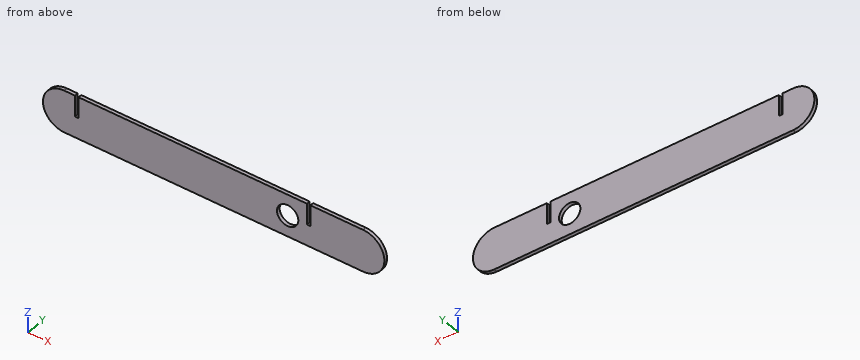
```python
from build123d import *

# Parameters (mm, degrees)
F0_R     = 4.7625
F1_DEPTH = 1.5875


with BuildPart() as f1:
    # F0 (on Front) → F1 (new body)
    with BuildSketch(Plane.XZ):
        with BuildLine():
            Line((-66.675, -9.525), (66.675, -9.525))
            ThreePointArc((66.675, -9.525), (76.2, 0), (66.675, 9.525))
            Line((66.675, 9.525), (43.18, 9.525))
            Line((43.18, 9.525), (43.18, 0))
            Line((43.18, 0), (41.5925, 0))
            Line((41.5925, 0), (41.5925, 9.525))
            Line((41.5925, 9.525), (-60.325, 9.525))
            Line((-60.325, 9.525), (-60.325, 0))
            Line((-60.325, 0), (-61.9125, 0))
            Line((-61.9125, 0), (-61.9125, 9.525))
            Line((-61.9125, 9.525), (-66.675, 9.525))
            ThreePointArc((-66.675, 9.525), (-76.2, 0), (-66.675, -9.525))
        make_face()
        with Locations((33.02, 0)):
            Circle(F0_R, mode=Mode.SUBTRACT)
    extrude(amount=F1_DEPTH)


solid = f1.part
```
Geometry check sheet. Reference: the model listing, model coordinates, mm. Give positions to 0.01 mm unless a question says otherwise; leave off trailing zeros. Write each loop counter-clockwise with the first axis right and the second up, starting at its lowest first coordinate (ties: lowest second). Pieces come first, ordered by that corner, then holes. Notation, with made-up numbers: (83.25, 4) -> (114.25, 4) arc R32 cw to (114.25, 43) -> close; hole circle Ø10 at (12, 46). An arc over 180 degrees is marked (long way). One line per question, with ' | ' between items.
Item 1: Depth check by flat-ended pin: pin 1 (0.8 mm diameter, centred on y = -1, z = 4, fed in from -X); pin 2 (6 mm diameter, centred on x = -16, z = -7.5, fed in from +Y); pin 3 (0.5 mm diameter, centred on x = -61, y = -0.5, fed in from +Z); pin 4 (0.8 mm diameter, centred on y = -0.5, z = 3.5, fed in from +X). Enter the tip coordinate at first touch or a pass-through.
Determined:
pin 1: x = -75.49 | pin 2: y = 0 | pin 3: z = 0 | pin 4: x = 75.68
Item 2: Sectioned sample at D-D, the plane z = 8.25. Record the boundary of the cut face in (x, y) (1 decimal), plus the area to 3 significant figures.
Determined:
outline: (-71.4, -1.6) -> (-61.9, -1.6) -> (-61.9, 0) -> (-71.4, 0) -> close; (-60.3, -1.6) -> (41.6, -1.6) -> (41.6, 0) -> (-60.3, 0) -> close; (43.2, -1.6) -> (71.4, -1.6) -> (71.4, 0) -> (43.2, 0) -> close | area: 222 mm^2
Item 3: Sectioned sample at B-B, the plane z = 2.5. Record the boundary of the cut face in (x, y) (1 decimal), plus the area to 3 significant figures.
Determined:
outline: (-75.9, -1.6) -> (-61.9, -1.6) -> (-61.9, 0) -> (-75.9, 0) -> close; (-60.3, -1.6) -> (29, -1.6) -> (29, 0) -> (-60.3, 0) -> close; (37.1, -1.6) -> (41.6, -1.6) -> (41.6, 0) -> (37.1, 0) -> close; (43.2, -1.6) -> (75.9, -1.6) -> (75.9, 0) -> (43.2, 0) -> close | area: 223 mm^2
Item 4: Sectioned sample at C-C, the plane x = 33.02. Record the boundary of the cut face in (y, z) (1 decimal).
Determined:
outline: (-1.6, -9.5) -> (0, -9.5) -> (0, -4.8) -> (-1.6, -4.8) -> close; (-1.6, 4.8) -> (0, 4.8) -> (0, 9.5) -> (-1.6, 9.5) -> close
Item 5: Scan lines: line 1 along Z through (x, y) = (33.02, -1.15) (1 decimal); line 2 along X through (y, z) = (-0.1, -0.5); line 3 along X through (y, z) = (-1, 3.25) (1 decimal). Record each from-to range of solid material in increasing order.
Determined:
line 1: -9.5 to -4.8, 4.8 to 9.5 | line 2: -76.19 to 28.28, 37.76 to 76.19 | line 3: -75.6 to -61.9, -60.3 to 29.5, 36.5 to 41.6, 43.2 to 75.6
